```python
from build123d import *

# Parameters (mm, degrees)
SKETCH1_W                = 68.1
SKETCH1_H                = 110
SKETCH1_R                = 2.1
SKETCH1_R_2              = 4.05
SKETCH1_R_3              = 1.6
BOSS_EXTRUDE1_DEPTH      = 7.7
SKETCH2_R                = 7.334333348
SKETCH2_R_2              = 11.073656437
BOSS_EXTRUDE2_DEPTH      = 5
SKETCH3_R                = 4.05
SKETCH3_R_2              = 3.2
CUT_EXTRUDE1_DEPTH       = 4
SKETCH4_W                = 68.1
SKETCH4_H                = 5
BOSS_EXTRUDE3_DEPTH      = 7.7
BOSS_EXTRUDE3_DEPTH_BACK = 7.7
BOSS_EXTRUDE4_DEPTH      = 115
SKETCH8_W                = 94.544818424
SKETCH8_H                = 30.580965824
CUT_EXTRUDE2_DEPTH       = 10
SKETCH9_W                = 3
SKETCH9_H                = 10
CUT_EXTRUDE3_DEPTH       = 79.1


with BuildPart() as part:
    # Sketch1 → Boss-Extrude1 (new body)
    with BuildSketch(Plane.XY):
        Rectangle(SKETCH1_W, SKETCH1_H)
        with Locations((20, 45)):
            Circle(SKETCH1_R, mode=Mode.SUBTRACT)
        with Locations((-20, 45)):
            Circle(SKETCH1_R, mode=Mode.SUBTRACT)
        with Locations((20, -45)):
            Circle(SKETCH1_R, mode=Mode.SUBTRACT)
        with Locations((-20, -45)):
            Circle(SKETCH1_R, mode=Mode.SUBTRACT)
        with Locations((0, 25)):
            Circle(SKETCH1_R_2, mode=Mode.SUBTRACT)
        with Locations((0, -25)):
            Circle(SKETCH1_R_2, mode=Mode.SUBTRACT)
        with Locations((0, 45)):
            Circle(SKETCH1_R_3, mode=Mode.SUBTRACT)
        with Locations((0, -45)):
            Circle(SKETCH1_R_3, mode=Mode.SUBTRACT)
    extrude(amount=BOSS_EXTRUDE1_DEPTH)

    # Sketch2 → Boss-Extrude2 (add)
    with BuildSketch(Plane(origin=(0, 0, 0), x_dir=(-1, 0, 0), z_dir=(0, 0, -1))):
        with Locations((0, 25)):
            Circle(SKETCH2_R)
        with Locations((0, -25)):
            Circle(SKETCH2_R_2)
    extrude(amount=-BOSS_EXTRUDE2_DEPTH)

    # Sketch3 → Cut-Extrude1 (cut)
    with BuildSketch(Plane(origin=(0, 0, 7.7), x_dir=(-1, 0, 0), z_dir=(0, 0, -1))):
        with Locations((-20, 45)):
            Circle(SKETCH3_R)
        with Locations((20, 45)):
            Circle(SKETCH3_R)
        with Locations((-20, -45)):
            Circle(SKETCH3_R)
        with Locations((20, -45)):
            Circle(SKETCH3_R)
        with Locations((0, 45)):
            Circle(SKETCH3_R_2)
        with Locations((0, -45)):
            Circle(SKETCH3_R_2)
    extrude(amount=CUT_EXTRUDE1_DEPTH, mode=Mode.SUBTRACT)

    # Sketch4 → Boss-Extrude3 (add, two sides)
    with BuildSketch(Plane.XY.offset(7.7)) as boss_extrude3_sk:
        with Locations((0, 57.5)):
            Rectangle(SKETCH4_W, SKETCH4_H)
    extrude(amount=BOSS_EXTRUDE3_DEPTH)
    extrude(boss_extrude3_sk.sketch, amount=-BOSS_EXTRUDE3_DEPTH_BACK)

    # Sketch7 → Boss-Extrude4 (add)
    with BuildSketch(Plane.XZ.offset(55)):
        Polygon((-34.05, 15.4), (-32.05, 15.4), (-34.05, 13.4), (-34.05, 0), (-39.05, 0), (-39.05, 15.4), align=None)
        Polygon((39.05, 0), (34.05, 0), (34.05, 13.4), (32.05, 15.4), (34.05, 15.4), (39.05, 15.4), align=None)
    extrude(amount=-BOSS_EXTRUDE4_DEPTH)

    # Sketch8 → Cut-Extrude2 (cut)
    with BuildSketch(Plane.XZ.offset(-55)):
        with Locations((-0.280192095, 7.459835347)):
            Rectangle(SKETCH8_W, SKETCH8_H)
    extrude(amount=-CUT_EXTRUDE2_DEPTH, mode=Mode.SUBTRACT)

    # Sketch9 → Cut-Extrude3 (cut, through all)
    with BuildSketch(Plane.ZY.offset(39.05)):
        with Locations((11.55, 0)):
            Rectangle(SKETCH9_W, SKETCH9_H)
        with Locations((11.55, 34.9)):
            Rectangle(SKETCH9_W, SKETCH9_H)
        with Locations((11.55, -34.9)):
            Rectangle(SKETCH9_W, SKETCH9_H)
    extrude(amount=-CUT_EXTRUDE3_DEPTH, mode=Mode.SUBTRACT)


solid = part.part
```
Geometry check sheet. Reference: the model listing, model coordinates, mm. A direction names the side the tool comes from. Give positions to 0.01 mm unless a question says otherwise; leave off trailing zeros. Order: outer loops, then holes, each group sorted by start corner. A loop starts at its lowest first (then second) coordinate and runs counter-clockwise, first axis right, second up. Notation, with made-up numbers: (6, 24.5) - (28, 24.5) arc R21 cw to (28, 44.5) - close; hole circle Ø4 at (12, -4.5). An arc over 180 degrees is marked (long way). Answer in a Markdown table with one row per item. Add a question column.
Q1. Cross-section at C-C, the plane y = -25. Enter the section's corners in (x, z), then the cut area to 4 significant figures.
Q2. Cross-section at B-B, the plane x = -20. Enter the section's corners in (y, z).
Q3. Cross-section at A-A, the plane y = -45. Count the separate pieces of the cut face and the enclosed holes in it, then the cut area to 3 significant figures.
Q4. Gauge pin test, flat ends, axial feed: pin 1 (5.5 mm diameter, centred on x = 20, y = -45, fed in from +Z); pin 2 (6 mm diameter, centred on x = -4.5, y = 36.5, fed in from +Z). Record the tip position at first contact, or that the pin passes through.
Q5. Mould release check, pull along Z, two halves, no side actions. Record for faces 4 (the flat face through (0, -25, 5)), 5 (the cylindrical face through (0.417, 48.173, 5.728)), 6 (the flat face through (-37, -5, 12)): pulls with the +Z half, pulls with the -Z half, needs draft (parallel to the pull), parting line crosses it, or undercut.
Q6. Tool access check on faces 1 (the flat face through (37, 35, 10.05)), 2 (the cylindrical face through (-19.473, 49.016, 5.728)), 3 (the flat face through (-34.05, -1, 9)). Record the directions out of +Z, -Z, +X, -X, +Y, -Y that give a thin tool (end or side, any length) a straight path to the whole face; none if there is none.
Q7. Cross-section at D-D, the plane y = 37.5. Enter the section's corners in (x, z), then the cut area to 3 significant figures.
Q8. Material ranges on probe 1 along X at (y, z) = (45, 0.9); probe 2 along Y at (x, z) = (20, 2.2); probe 3 along Y at (x, z) = (-20, 4.85), recorded low to high. Write a range as from..to.
Check values:
| question | item | result |
|---|---|---|
| 1 | outline | (-39.05, 0) - (39.05, 0) - (39.05, 15.4) - (32.05, 15.4) - (34.05, 13.4) - (34.05, 7.7) - (4.05, 7.7) - (4.05, 5) - (-4.05, 5) - (-4.05, 7.7) - (-34.05, 7.7) - (-34.05, 13.4) - (-32.05, 15.4) - (-39.05, 15.4) - close |
| 1 | area | 660.5 mm^2 |
| 2 | outline | (-55, 0) - (-47.1, 0) - (-47.1, 3.7) - (-49.05, 3.7) - (-49.05, 7.7) - (-55, 7.7) - close; (-42.9, 0) - (42.9, 0) - (42.9, 3.7) - (40.95, 3.7) - (40.95, 7.7) - (-40.95, 7.7) - (-40.95, 3.7) - (-42.9, 3.7) - close; (47.1, 0) - (55, 0) - (55, 7.7) - (49.05, 7.7) - (49.05, 3.7) - (47.1, 3.7) - close |
| 3 | separate pieces | 4 |
| 3 | enclosed holes | 0 |
| 3 | area | 549 mm^2 |
| 4 | pin 1 | stops at z = 3.7 |
| 4 | pin 2 | stops at z = 7.7 |
| 5 | face 4 | pulls with the +Z half |
| 5 | face 5 | needs draft |
| 5 | face 6 | undercut |
| 6 | face 1 | +X, -X |
| 6 | face 2 | +Z |
| 6 | face 3 | +Y, -Y |
| 7 | outline | (-39.05, 0) - (39.05, 0) - (39.05, 10.05) - (34.05, 10.05) - (34.05, 7.7) - (-34.05, 7.7) - (-34.05, 10.05) - (-39.05, 10.05) - close; (-39.05, 13.05) - (-34.05, 13.05) - (-34.05, 13.4) - (-32.05, 15.4) - (-39.05, 15.4) - close; (32.05, 15.4) - (34.05, 13.4) - (34.05, 13.05) - (39.05, 13.05) - (39.05, 15.4) - close |
| 7 | area | 652 mm^2 |
| 8 | probe 1 | x = -39.05..-22.1, -17.9..-1.6, 1.6..17.9, 22.1..39.05 |
| 8 | probe 2 | y = -55..-47.1, -42.9..42.9, 47.1..55 |
| 8 | probe 3 | y = -55..-49.05, -40.95..40.95, 49.05..55 |
